CAD build for the part. Positions are in the model's coordinates, mm. Face numbers are marked on the shaded views. Round coordinates to 2 decimals unless told otherwise and drop trailing zeros. Loops run counter-clockwise (first coordinate to the right, second up) from the corner with the lowest first, then second, coordinate; pieces in that order, holes last. Notation, with made-up numbers: (71, 3) - (96, 3) arc R30 ccw to (96, 25) - close; hole circle Ø1 at (64, 40.25). An arc over 180 degrees is marked (long way). Use one line per item in the form item = value.
from build123d import *

# Parameters (mm, degrees)
SKETCH2_R           = 38.1
BOSS_EXTRUDE1_DEPTH = 279.4
BOSS_EXTRUDE2_DEPTH = 25.4


with BuildPart() as part:
    # Sketch2 → Boss-Extrude1 (new body)
    with BuildSketch(Plane(origin=(0, 0, 0), x_dir=(0, 0, -1), z_dir=(1, 0, 0))):
        Circle(SKETCH2_R)
    boss_extrude1 = extrude(amount=BOSS_EXTRUDE1_DEPTH)

    # Sketch3 → Boss-Extrude2 (add)
    with BuildSketch(Plane(origin=(279.4, 0, 0), x_dir=(0, 0, -1), z_dir=(1, 0, 0))):
        with BuildLine():
            Line((-38.1, 0), (-38.1, 203.2))
            Line((-38.1, 203.2), (38.1, 203.2))
            Line((38.1, 203.2), (38.1, 0))
            ThreePointArc((38.1, 0), (0, -38.1), (-38.1, 0))
        make_face()
    boss_extrude2 = extrude(amount=BOSS_EXTRUDE2_DEPTH)

    # Mirror1: Boss-Extrude1, Boss-Extrude2 across plane
    add(boss_extrude1.mirror(Plane(origin=(0, 0, 0), x_dir=(0, 0, 1), z_dir=(1, 0, 0))))
    add(boss_extrude2.mirror(Plane(origin=(0, 0, 0), x_dir=(0, 0, 1), z_dir=(1, 0, 0))))


solid = part.part
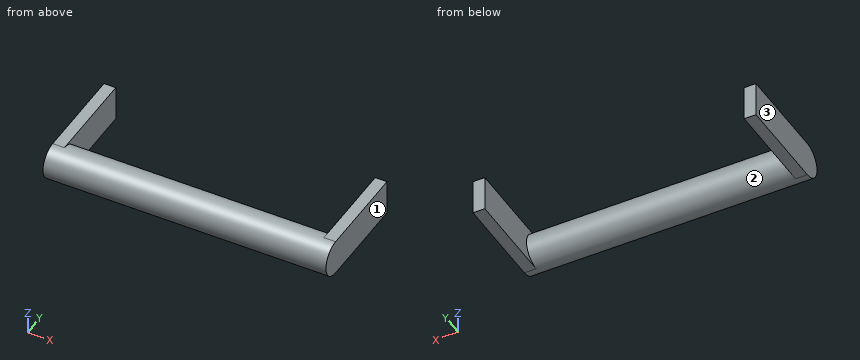
1) Slice it at C-C (x = -15). Write the cut outline in (y, z).
Report:
outline = circle Ø76.2 at (0, 0)
2) Slice it at A-A (y = 105). Write the cut outline in (x, z), plus the area to 3 significant figures.
Report:
outline = (-304.8, -38.1) - (-279.4, -38.1) - (-279.4, 38.1) - (-304.8, 38.1) - close; (279.4, -38.1) - (304.8, -38.1) - (304.8, 38.1) - (279.4, 38.1) - close
area = 3,870 mm^2
3) Flat gauge pins, fed straight in: pin 1 (8 mm diameter, centred on x = -29, y = 35, fed in from +Z); pin 2 (1 mm diameter, centred on x = -137, z = -17, fed in from +Y); pin 3 (6 mm diameter, centred on x = 158, y = 11.5, fed in from +Z). Where does each tip first touch, or does it go through?
Report:
pin_1 = 22.15
pin_2 = 34.34
pin_3 = 37.14
4) Drill centre lines: probe 1 along X at (y, z) = (114, 24.5); probe 2 along Y at (x, z) = (-46.5, -1); probe 3 along Y at (x, z) = (-269.5, -3). Where is each one in solid material? Low to high.
Report:
probe_1 = -304.8 to -279.4, 279.4 to 304.8
probe_2 = -38.09 to 38.09
probe_3 = -37.98 to 37.98
5) Slice it at B-B (z = 0). Write the cut outline in (x, y).
Report:
outline = (-304.8, -38.1) - (304.8, -38.1) - (304.8, 203.2) - (279.4, 203.2) - (279.4, 38.1) - (-279.4, 38.1) - (-279.4, 203.2) - (-304.8, 203.2) - close
6) Slice it at D-D (y = 10). Write the cut outline in (x, z), plus the area to 3 significant figures.
Report:
outline = (-304.8, -38.1) - (-279.4, -38.1) - (-279.4, -36.76) - (279.4, -36.76) - (279.4, -38.1) - (304.8, -38.1) - (304.8, 38.1) - (279.4, 38.1) - (279.4, 36.76) - (-279.4, 36.76) - (-279.4, 38.1) - (-304.8, 38.1) - close
area = 45,000 mm^2
7) Two-plate mould, pull along X, no slides. Class the marked faces 1, 2 and 3: +X half, -X half, draft (parallel to the pull), parting line (faces both ways), or undercut.
Report:
face_1 = +X half
face_2 = undercut
face_3 = -X half
